Check sheet for the modelled part. Datum: model origin and axes. Units: mm. Face numbers are marked on the shaded views. A direction names the side the tool comes from. Round coordinates to 2 decimals unless told otherwise and drop trailing zeros. Loops run counter-clockwise (first coordinate to the right, second up) from the corner with the lowest first, then second, coordinate; pieces in that order, holes last. Notation, with made-up numbers: (71.25, 89.25) -> (113.25, 89.25) arc R16 cw to (113.25, 108.25) -> close; hole circle Ø6 at (66, 64.5). An arc over 180 degrees is marked (long way). One line per item, written item: value. Start each with the question number.
1. Cross-section at B-B on z = 5. Record the cut outline in (x, y).
2. Cross-section at C-C on x = -1.5. Record the cut outline in (y, z) (3 decimals).
3. Go/stop test with flat-tipped pins: pin 1 (0.5 mm diameter, centred on x = 1.5, z = 1.5, fed in from -Y); pin 2 (4.5 mm diameter, centred on y = -0.5, z = 5, fed in from +X); pin 3 (2.5 mm diameter, centred on y = 0, z = 4.572, fed in from -X); pin 4 (4 mm diameter, centred on x = 6.5, z = 6.5, fed in from +Y). Record where each tip stops, or that it passes through.
4. Cross-section at D-D on y = 3.5. Record the cut outline in (x, z) (3 decimals).
5. Set-up check for the marked faces 5 and 6: record each of +Z, -Z, +X, -X, +Y, -Y from which the full face is reachable in a straight line by a thin tool's end or side.
6. Cross-section at A-A on z = 1. Record the cut outline in (x, y).
7. Material ranges on L1, parallel to Z at x = -1.35, y = 0; L2, parallel to X at y = -0.75, z = 6.25; L3, parallel to Z at x = 8.5, y = 2.75, recorded low to high.
8. Release check for a two-part mould opening along X. For the marked faces 1, 2, 3 and 4 record: +X half, -X half, draft (parallel to the pull), parting line (faces both ways), or undercut.
from build123d import *

# Parameters (mm, degrees)
F0_R     = 1.016
F1_DEPTH = 2.667
F2_W     = 19.05
F2_H     = 19.05
F3_DEPTH = 0.762
F4_W     = 2.1082
F4_H     = 12.7
F5_DEPTH = 12.7
F6_R     = 5.08


with BuildPart() as f1:
    # F0 (on Right) → F1 (new body, symmetric)
    with BuildSketch(Plane.YZ):
        with BuildLine():
            Line((-2.85, 4.77), (-2.85, 0))
            Line((-2.85, 0), (2.85, 0))
            Line((2.85, 0), (2.85, 4.77))
            ThreePointArc((2.85, 4.77), (2.015254, 6.785254), (0, 7.62))
            ThreePointArc((0, 7.62), (-2.015254, 6.785254), (-2.85, 4.77))
        make_face()
        with Locations((0, 4.572)):
            Circle(F0_R, mode=Mode.SUBTRACT)
    extrude(amount=F1_DEPTH, both=True)

    # F2 (on face) → F3 (join)
    with BuildSketch(Plane(origin=(0, 0, 0), x_dir=(1, 0, 0), z_dir=(0, 0, -1))):
        Rectangle(F2_W, F2_H)
    extrude(amount=F3_DEPTH)

    # F4 (on Front) → F5 (cut, symmetric)
    with BuildSketch(Plane.XZ):
        with Locations((0, 6.35)):
            Rectangle(F4_W, F4_H)
    extrude(amount=F5_DEPTH, both=True, mode=Mode.SUBTRACT)

    # F6
    f6_edges = [f1.edges().sort_by_distance(p)[0] for p in [
        (9.525, 9.525, -0.381),
        (-9.525, 9.525, -0.381),
        (9.525, -9.525, -0.381),
        (-9.525, -9.525, -0.381),
    ]]
    fillet(f6_edges, radius=F6_R)


solid = f1.part
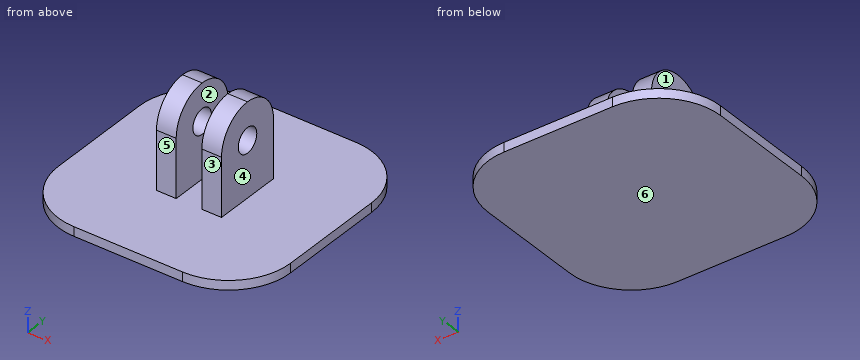
Taken from the geometry:
1. outline: (-2.67, -2.84) -> (-1.05, -2.84) -> (-1.05, -0.92) -> (-2.67, -0.92) -> close; (-2.67, 0.92) -> (-1.05, 0.92) -> (-1.05, 2.84) -> (-2.67, 2.84) -> close; (1.05, -2.84) -> (2.67, -2.84) -> (2.67, -0.92) -> (1.05, -0.92) -> close; (1.05, 0.92) -> (2.67, 0.92) -> (2.67, 2.84) -> (1.05, 2.84) -> close
2. outline: (-9.525, -0.762) -> (9.525, -0.762) -> (9.525, 0) -> (2.85, 0) -> (2.85, 4.77) arc R2.85 ccw to (0, 7.62) arc R2.85 ccw to (-2.85, 4.77) -> (-2.85, 0) -> (-9.525, 0) -> close; hole circle Ø2.032 at (0, 4.572)
3. pin 1: stops at y = -2.85
3. pin 2: stops at x = 2.67
3. pin 3: stops at x = -2.67
3. pin 4: passes through
4. outline: (-9.525, -0.762) -> (9.525, -0.762) -> (9.525, 0) -> (-9.525, 0) -> close
5. face 5: +Z, +X, -X, -Y
5. face 6: -Z, +X, -X, +Y, -Y
6. outline: (-2.67, -2.85) -> (-1.05, -2.85) -> (-1.05, 2.85) -> (-2.67, 2.85) -> close; (1.05, -2.85) -> (2.67, -2.85) -> (2.67, 2.85) -> (1.05, 2.85) -> close
7. L1: z = -0.76 to 3.56, 5.59 to 7.62
7. L2: x = -2.67 to -1.05, 1.05 to 2.67
7. L3: z = -0.76 to 0
8. face 1: -X half
8. face 2: undercut
8. face 3: draft
8. face 4: +X half
